Work out the finished part from the listing and answer in its coordinate system (mm). A direction names the side the tool comes from. Coordinates: 2 decimals unless noted, no trailing zeros. Order: outer loops, then holes, each group sorted by start corner. A loop starts at its lowest first (then second) coordinate and runs counter-clockwise, first axis right, second up. Notation, with made-up numbers: M 62,-7 L 99,-7 A25 cw 99,19 Z; hole C 47,5.25 d9. An arc over 180 degrees is marked long. Use a Markdown table: item, result.
from build123d import *

# Parameters (mm, degrees)
BOSS_EXTRUDE1_DEPTH     = 20
SKETCH3_R               = 0.95
CUT_EXTRUDE1_DEPTH      = 5
CUT_EXTRUDE2_DEPTH      = 23.837378659
CUT_EXTRUDE2_DEPTH_BACK = 23.837378659
SKETCH4_R               = 0.975


with BuildPart() as part:
    # Sketch2 → Boss-Extrude1 (new body)
    with BuildSketch(Plane.XY):
        Polygon((-1.080060634, 2.442708333), (2.419939366, 2.442708333), (2.419939366, -2.657291667), (4.419939366, -2.657291667), (4.419939366, -7.657291667), (-3.080060634, -7.657291667), (-3.080060634, -2.657291667), (-1.080060634, -2.657291667), align=None)
    extrude(amount=BOSS_EXTRUDE1_DEPTH)

    # Sketch3 → Cut-Extrude1 (cut)
    with BuildSketch(Plane.XY.offset(20)):
        with Locations((0.669939366, -2.757291667)):
            Circle(SKETCH3_R)
    extrude(amount=-CUT_EXTRUDE1_DEPTH, mode=Mode.SUBTRACT)

    # Sketch4 → Cut-Extrude2 (cut, two sides: drawn at the far end of the back side and taken through both)
    with BuildSketch(Plane(origin=(0, 2.442708333, 0), x_dir=(1, 0, 0), z_dir=(0, 1, 0)).offset(-CUT_EXTRUDE2_DEPTH_BACK)):
        with Locations(Location((0.669939366, -8.322927776, 0), (0, 0, 270))):
            Circle(SKETCH4_R)
        with Locations((0.669939366, 0.86)):
            Circle(SKETCH4_R)
    extrude(amount=CUT_EXTRUDE2_DEPTH + CUT_EXTRUDE2_DEPTH_BACK, mode=Mode.SUBTRACT)


solid = part.part
(1) A cutting plane is placed at A-A (x = 0). Determine the outline of the cut face in (y, z).
Conclusion:
| item | result |
|---|---|
| outline | M -7.66,0 L 2.44,0 L 2.44,7.61 L -7.66,7.61 Z; M -7.66,9.03 L 2.44,9.03 L 2.44,20 L -2.08,20 L -2.08,15 L -3.43,15 L -3.43,20 L -7.66,20 Z |
(2) Determine the mould class of faces 1 (the flat face through (-1.08, 0, 10)), 2 (the flat face through (1, 2.443, 10)), 3 (the flat face through (1, -3, 15)) for opening direction Y: pulls with the +Y half, pulls with the -Y half, needs draft (parallel to the pull), parting line crosses it, or undercut.
Conclusion:
| item | result |
|---|---|
| face 1 | needs draft |
| face 2 | pulls with the +Y half |
| face 3 | undercut |
(3) A cutting plane is placed at D-D (z = 16). Determine the outline of the cut face in (x, y).
Conclusion:
| item | result |
|---|---|
| outline | M -3.08,-7.66 L 4.42,-7.66 L 4.42,-2.66 L 2.42,-2.66 L 2.42,2.44 L -1.08,2.44 L -1.08,-2.66 L -3.08,-2.66 Z; hole C 0.67,-2.76 d1.9 |
(4) A cutting plane is placed at C-C (z = 6.75). Determine the outline of the cut face in (x, y), then the cut area to 4 significant figures.
Conclusion:
| item | result |
|---|---|
| outline | M -3.08,-7.66 L 4.42,-7.66 L 4.42,-2.66 L 2.42,-2.66 L 2.42,2.44 L -1.08,2.44 L -1.08,-2.66 L -3.08,-2.66 Z |
| area | 55.35 mm2 |
(5) Straight lines are drawn through the part: L1, parallel to Z at x = 0.75, y = 0.5; L2, parallel to X at y = -2.5, z = 2; L3, parallel to Y at x = -1.25, z = 15.5. For each, find the intervals that lie inside material, in ascending order.
Conclusion:
| item | result |
|---|---|
| L1 | 0.11 to 7.35, 9.29 to 20 |
| L2 | -1.08 to 2.42 |
| L3 | -7.66 to -2.66 |
(6) Given P1, Ø1, axis at x = -2, z = 11.5, coming from the +Y side, flat-ended and moving along its own axis, determine where the tip first touches the part or whether it passes through.
Conclusion:
| item | result |
|---|---|
| P1 | y = -2.66 |
(7) Which of the six approach directions +Z, -Z, +X, -X, +Y, -Y give full straight-line access (tool end or side, diameter ignored) to faces 4 (the flat face through (2.42, 0, 10)), 5 (the cylindrical face through (0.963, -2.678, 9.253)), 6 (the flat face through (-2, -2.657, 10)), 7 (the cylindrical face through (-0.08, -3.34, 17.54))?
Conclusion:
| item | result |
|---|---|
| face 4 | +Z, -Z, +X, +Y |
| face 5 | +Y, -Y |
| face 6 | +Z, -Z, -X, +Y |
| face 7 | +Z |
(8) A cutting plane is placed at B-B (y = 0.75). Determine the outline of the cut face in (x, z) (3 decimals).
Conclusion:
| item | result |
|---|---|
| outline | M -1.08,0 L 0.211,0 A0.975 cw 1.129,0 L 2.42,0 L 2.42,20 L -1.08,20 Z; hole C 0.67,8.323 d1.95 |
